from build123d import *

# Parameters (mm, degrees)
CORTAR_EXTRUIR3_DEPTH      = 8
CORTAR_EXTRUIR3_DEPTH_BACK = 27
CROQUIS5_R                 = 7.9375
CROQUIS9_R                 = 3.175
CORTAR_EXTRUIR5_DEPTH      = 18
CROQUIS10_R                = 4.765
CORTAR_EXTRUIR6_DEPTH      = 35
CROQUIS11_R                = 35
SALIENTE_EXTRUIR1_DEPTH    = 14.24
CROQUIS13_R                = 8.035449209
CORTAR_EXTRUIR8_DEPTH      = 30.21


with BuildPart() as part:
    # Croquis1 → Revolución3 (revolve)
    with BuildSketch(Plane.XY, mode=Mode.PRIVATE) as revoluci_n3_sk:
        with BuildLine():
            Line((0, 43.044568245), (30, 43.044568245))
            Line((30, 43.044568245), (30, 20.044568245))
            Line((30, 20.044568245), (12.985796912, 20.044568245))
            Line((12.985796912, 20.044568245), (12.985796912, 10.406207601))
            ThreePointArc((12.985796912, 10.406207601), (13.175212613, 9.391052882), (13.717969076, 8.512512712))
            Line((13.717969076, 8.512512712), (32.309744815, 5.485961945))
            ThreePointArc((32.309744815, 5.485961945), (33.884795273, 4.831882369), (35, 3.541563627))
            Line((35, 3.541563627), (35, -0.490098714))
            Line((35, -0.490098714), (13.468735488, -0.490098714))
            Line((13.468735488, -0.490098714), (13.468735488, -18.538757946))
            Line((13.468735488, -18.538757946), (31.979226627, -20.513196287))
            ThreePointArc((31.979226627, -20.513196287), (33.927671218, -21.380602851), (35, -23.224224681))
            Line((35, -23.224224681), (35, -35.501069654))
            Line((35, -35.501069654), (24.334695592, -35.501069654))
            Line((24.334695592, -35.501069654), (24.334695592, -43.520130292))
            Line((24.334695592, -43.520130292), (34.538342083, -43.520130292))
            Line((34.538342083, -43.520130292), (34.538342083, -52.477142798))
            Line((34.538342083, -52.477142798), (24.334695592, -52.477142798))
            Line((24.334695592, -52.477142798), (24.334695592, -58.946096275))
            Line((24.334695592, -58.946096275), (34.538342083, -58.946096275))
            Line((34.538342083, -58.946096275), (34.538342083, -64.917437946))
            Line((34.538342083, -64.917437946), (24.334695592, -64.917437946))
            Line((24.334695592, -64.917437946), (24.334695592, -72.132809132))
            Line((24.334695592, -72.132809132), (34.538342083, -72.132809132))
            Line((34.538342083, -72.132809132), (34.538342083, -77.357733094))
            Line((34.538342083, -77.357733094), (24.334695592, -77.357733094))
            Line((24.334695592, -77.357733094), (24.334695592, -104.221668074))
            Line((24.334695592, -104.221668074), (34.538342083, -104.221668074))
            ThreePointArc((34.538342083, -104.221668074), (34.864783527, -104.356884547), (35, -104.683325991))
            Line((35, -104.683325991), (35, -120.950877143))
            ThreePointArc((35, -120.950877143), (34.933442046, -121.487214162), (34.737806004, -121.991013624))
            Line((34.737806004, -121.991013624), (0, -121.955431755))
            Line((0, -121.955431755), (0, 43.044568245))
        make_face()
    revolve(revoluci_n3_sk.sketch.rotate(Axis((0, 43.044568245, 0), (0, -1, 0)), 180), axis=Axis((0, 43.044568245, 0), (0, -1, 0)))

    # Croquis5 → Cortar-Extruir3 (cut, two sides: drawn at the far end of the back side and taken through both)
    with BuildSketch(Plane(origin=(0, -104.221668074, 0), x_dir=(1, 0, 0), z_dir=(0, 1, 0)).offset(-CORTAR_EXTRUIR3_DEPTH_BACK)):
        with Locations(Location((0.097949209, 0, 0), (0, 0, 270))):
            Circle(CROQUIS5_R)
    extrude(amount=CORTAR_EXTRUIR3_DEPTH + CORTAR_EXTRUIR3_DEPTH_BACK, mode=Mode.SUBTRACT)

    # Croquis9 → Cortar-Extruir5 (cut)
    with BuildSketch(Plane(origin=(0, 43.044568245, 0), x_dir=(1, 0, 0), z_dir=(0, 1, 0))):
        with Locations(Location((0, 23, 0), (0, 0, 180))):
            Circle(CROQUIS9_R)
        with Locations(Location((0, -23, 0), (0, 0, 180))):
            Circle(CROQUIS9_R)
    extrude(amount=-CORTAR_EXTRUIR5_DEPTH, mode=Mode.SUBTRACT)

    # Croquis10 → Cortar-Extruir6 (cut)
    with BuildSketch(Plane(origin=(0, 43.044568245, 0), x_dir=(1, 0, 0), z_dir=(0, 1, 0))):
        with Locations(Location((0, 0, 0), (0, 0, 180))):
            Circle(CROQUIS10_R)
    extrude(amount=-CORTAR_EXTRUIR6_DEPTH, mode=Mode.SUBTRACT)

    # Croquis11 → Saliente-Extruir1 (add)
    with BuildSketch(Plane(origin=(0, -104.221668074, 0), x_dir=(1, 0, 0), z_dir=(0, 1, 0))):
        with Locations(Location((0, 0, 0), (0, 0, 180))):
            Circle(CROQUIS11_R)
    extrude(amount=SALIENTE_EXTRUIR1_DEPTH)

    # Croquis13 → Cortar-Extruir8 (cut)
    with BuildSketch(Plane.XZ.offset(104.221668074)):
        Circle(CROQUIS13_R)
    extrude(amount=-CORTAR_EXTRUIR8_DEPTH, mode=Mode.SUBTRACT)


solid = part.part
Input: part model. Units: mm. Frame: model coordinates. A direction names the side the tool comes from. Coordinates: 2 decimals unless noted, no trailing zeros. Loops run counter-clockwise (first coordinate to the right, second up) from the corner with the lowest first, then second, coordinate; pieces in that order, holes last.
(1) Set-up query: faces 1 (the face through (-32.943, -61.974, -10.374)), 2 (the face through (-16.128, 31.384, -25.296)), 3 (the face through (7.587, -97.201, -34.168)). Return all of +Z, -Z, +X, -X, +Y, -Y with unobstructed straight access to the full face (end or side cutting, diameter ignored); none if empty.
(2) Section A-A on y = -82. Return the cut outline in (x, z).
(3) First-contact query: pin 1 Ø8 at (y, z) = (-35.5, -7) entering from +X; pin 2 Ø8 at (x, y) = (-10.5, -105) entering from +Z; pin 3 Ø3 at (x, z) = (-24.5, 24) entering from +Y. Flat tips, straight axial feed; report the tip coordinate or a pass-through.
(4) Section B-B on x = -19.5. Count the separate pieces of the cut face and the enclosed holes in it, then the cut area to 3 significant figures.
(5) Pull-direction query (Z, two-part tool) for faces 4 (the face through (7, -43.52, -24)), 5 (the face through (7.587, -29.449, 34.168)), 6 (the face through (0, 8.045, 0)); classes: released by +Z, released by -Z, zero draft, split by the parting line, or undercut.
(6) Material intervals for probe 1 along Y at (x, z) = (11.5, -8); probe 2 along Z at (x, y) = (0, 37) (3 decimals); probe 3 along Y at (x, z) = (-11, -13), sorted ascending.
Data:
1. face 1: none
1. face 2: +Y
1. face 3: +Y, -Y
2. outline: circle Ø48.67 at (0, 0); hole circle Ø16.07 at (0, 0)
3. pin 1: stops at x = 34.87
3. pin 2: stops at z = 34.39
3. pin 3: stops at y = 5.37
4. separate pieces: 3
4. enclosed holes: 0
4. area: 6,380 mm2
5. face 4: zero draft
5. face 5: split by the parting line
5. face 6: undercut
6. probe 1: y = -121.97 to -18.6, -0.49 to 8.47, 20.04 to 43.04
6. probe 2: z = -30 to -26.175, -19.825 to -4.765, 4.765 to 19.825, 26.175 to 30
6. probe 3: y = -121.97 to -18.92, -0.49 to 7.97, 20.04 to 43.04
